Design review of the part built by this model. Coordinates are the model's own, in mm. A direction names the side the tool comes from. Give positions to 0.01 mm unless a question says otherwise; leave off trailing zeros. Answer as a JSON object with one key per item and string values.
```python
from build123d import *

# Parameters (mm, degrees)
SKETCH1_R           = 4.7625
BOSS_EXTRUDE1_DEPTH = 19.05
SKETCH2_R           = 3
CUT_EXTRUDE1_DEPTH  = 9.525
SKETCH3_R           = 3.175
CUT_EXTRUDE2_DEPTH  = 9.525
CUT_EXTRUDE3_REACH  = 11.525
SKETCH4_R           = 2.413


with BuildPart() as part:
    # Sketch1 → Boss-Extrude1 (new body)
    with BuildSketch(Plane(origin=(0, 0, 0), x_dir=(1, 0, 0), z_dir=(0, 1, 0))):
        Circle(SKETCH1_R)
    extrude(amount=BOSS_EXTRUDE1_DEPTH)

    # Sketch2 → Cut-Extrude1 (cut)
    with BuildSketch(Plane.XZ):
        Circle(SKETCH2_R)
    extrude(amount=-CUT_EXTRUDE1_DEPTH, mode=Mode.SUBTRACT)

    # Sketch3 → Cut-Extrude2 (cut)
    with BuildSketch(Plane(origin=(0, 19.05, 0), x_dir=(1, 0, 0), z_dir=(0, 1, 0))):
        Circle(SKETCH3_R)
    extrude(amount=-CUT_EXTRUDE2_DEPTH, mode=Mode.SUBTRACT)

    # Sketch4 → Cut-Extrude3 (cut, up to next)
    with BuildSketch(Plane(origin=(0, 0, -4.7625), x_dir=(-1, 0, 0), z_dir=(0, 0, -1)), mode=Mode.PRIVATE) as cut_extrude3_sk1:
        with Locations((0, 14.2875)):
            Circle(SKETCH4_R)
    cut_extrude3_tool1 = extrude(cut_extrude3_sk1.sketch, amount=-CUT_EXTRUDE3_REACH, mode=Mode.PRIVATE) & part.part
    add(cut_extrude3_tool1.solids().sort_by_distance((0, 14.2875, -4.7625))[0], mode=Mode.SUBTRACT)
    # Sketch4 → Cut-Extrude3 (cut, up to next)
    with BuildSketch(Plane(origin=(0, 0, -4.7625), x_dir=(-1, 0, 0), z_dir=(0, 0, -1)), mode=Mode.PRIVATE) as cut_extrude3_sk2:
        with Locations((0, 4.7625)):
            Circle(SKETCH4_R)
    cut_extrude3_tool2 = extrude(cut_extrude3_sk2.sketch, amount=-CUT_EXTRUDE3_REACH, mode=Mode.PRIVATE) & part.part
    add(cut_extrude3_tool2.solids().sort_by_distance((0, 4.7625, -4.7625))[0], mode=Mode.SUBTRACT)


solid = part.part
```
(1) For faces 4 (the cylindrical face through (-0.69, 14.35, 3.1)), 5 (the cylindrical face through (0, 5, 3)), 6 (the cylindrical face through (0.5, 2.4, -3.3)), list the 3-axis set-ups (+Z, -Z, +X, -X, +Y, -Y) from which the entire face can be reached by the end or side of a thin tool; tool diameter is ignored.
Here are the results:
{"face 4": "+Y", "face 5": "+Y, -Y", "face 6": "-Z"}
(2) The part is to be moulded in two halves that separate along X. For faces 1 (the cylindrical face through (-1.03, 9.39, 4.65)), 2 (the cylindrical face through (1.9, 12.8, -3.4)), 3 (the flat face through (1, 0, 3)), say which applies: +X half, -X half, draft (parallel to the pull), parting line (faces both ways), or undercut.
Here are the results:
{"face 1": "parting line", "face 2": "undercut", "face 3": "draft"}
(3) For line 1 along Y through (x, z) = (0, -3.95); line 2 along Y through (x, z) = (-1.25, -3.25); line 3 along X through (y, z) = (13.25, 1.5), list the stretches that pass through material, from the lowest coordinate up.
Here are the results:
{"line 1": "y = 0 to 2.35, 7.18 to 11.87, 16.7 to 19.05", "line 2": "y = 0 to 2.7, 6.83 to 12.22, 16.35 to 19.05", "line 3": "x = -4.52 to -2.8, 2.8 to 4.52"}
(4) We need section B-B, the plane x = 0. Give the number of separate pieces and of enclosed holes in the cut face, then the cut area to 3 significant figures.
Here are the results:
{"separate pieces": "4", "enclosed holes": "0", "area": "47.7 mm²"}
